Design review of the part built by this model. Coordinates are the model's own, in mm. A direction names the side the tool comes from. Give positions to 0.01 mm unless a question says otherwise; leave off trailing zeros. Order: outer loops, then holes, each group sorted by start corner. A loop starts at its lowest first (then second) coordinate and runs counter-clockwise, first axis right, second up. Notation, with made-up numbers: (-29.75, 77) -> (-23.75, 77) arc R11 cw to (-23.75, 85) -> close; hole circle Ø8 at (15.5, -34.75). An arc over 180 degrees is marked (long way). Use a Markdown table: item, result. Add a question column.
```python
from build123d import *

# Parameters (mm, degrees)
F1_DEPTH       = 250
F3_D           = 3.7973
F3_CSINK_D     = 7.7978
F3_CSINK_ANGLE = 82
F2_W           = 5
F2_H           = 110
F4_DEPTH       = 13.001
F5_R           = 4.99999
F6_T1_DEPTH    = 240.00002
F6_T6_ANGLE    = 359.64
F6_T12_ANGLE   = 359.64


# Not quite as in the source:
# - a fillet or chamfer that OpenCascade refuses, or shapes differently, is made with other operations: its cross-section is extruded or revolved along the edge and cut away or added
# - a fillet or chamfer is up to 0.001 mm smaller than in the source, because OpenCascade refuses the exact size


with BuildPart() as f1:
    # F0 (on Front) → F1 (new body)
    with BuildSketch(Plane.XZ):
        Polygon((-15, 13), (-25, 13), (-25, 0), (0, 0), (0, 3), (-15, 3), align=None)
    extrude(amount=F1_DEPTH)

    # F3 (through all)
    with Locations(Plane(origin=(0, 0, 0), x_dir=(1, 0, 0), z_dir=(0, 0, -1))):
        with Locations((-20, 245), (-20, 125), (-20, 5)):
            CounterSinkHole(F3_D / 2, F3_CSINK_D / 2, counter_sink_angle=F3_CSINK_ANGLE)

    # F2 (on face) → F4 (cut, through all)
    with BuildSketch(Plane(origin=(0, 0, 0), x_dir=(1, 0, 0), z_dir=(0, 0, -1))):
        with Locations((-22.5, 185)):
            Rectangle(F2_W, F2_H)
        with Locations((-22.5, 65)):
            Rectangle(F2_W, F2_H)
    extrude(amount=-F4_DEPTH, mode=Mode.SUBTRACT)

    # F5 (radius 5 in the source; OpenCascade refuses exactly that, so slightly less here)
    f5_edges = [f1.edges().sort_by_distance(p)[0] for p in [
        (-25, 0, 6.5),
        (-25, -10, 6.5),
        (-25, -120, 6.5),
        (-25, -130, 6.5),
        (-25, -240, 6.5),
        (-25, -250, 6.5),
        (-15, -250, 8),
        (0, -250, 1.5),
        (-15, 0, 8),
        (0, 0, 1.5),
    ]]
    fillet(f5_edges, radius=F5_R)

    # F6: chamfer of 4 x 10 on 1 edges, made by hand

    # F6_s2 → F6_t1 (join)
    with BuildSketch(Plane.XZ.offset(4.99999)):
        Polygon((-15, 7), (-5, 3), (-15, 3), align=None)
    extrude(amount=F6_T1_DEPTH)


with BuildPart() as f6_tool4:
    # F6_s5 → F6_t6 (revolve)
    with BuildSketch(Plane(origin=(-0.0322045944, -5.1254529469, 0), x_dir=(0, 0, 1), z_dir=(0.006283144, 0.9999802609, 0))):
        Polygon((7, -14.9681895603), (3, -4.9681895603), (3, -14.9681895603), align=None)
    revolve(axis=Axis((-19.99999, -4.99999, 3), (0, 0, -1)), revolution_arc=F6_T6_ANGLE)

    split(bisect_by=Plane.XZ, keep=Keep.TOP)

    split(bisect_by=Plane.YZ.offset(-20), keep=Keep.TOP)


with BuildPart() as f1_1:
    add(f1.part)

    # F6_t3: union F6_tool4
    add(f6_tool4.part)


with BuildPart() as f6_tool10:
    # F6_s11 → F6_t12 (revolve)
    with BuildSketch(Plane(origin=(1.538550391, -244.8646775786, 0), x_dir=(0, 0, 1), z_dir=(0.006283144, -0.9999802609, 0))):
        Polygon((7, 16.5389755517), (3, 6.5389755517), (3, 16.5389755517), align=None)
    revolve(axis=Axis((-19.99999, -245.00001, 3), (0, 0, 1)), revolution_arc=F6_T12_ANGLE)

    split(bisect_by=Plane.XZ.offset(250), keep=Keep.BOTTOM)

    split(bisect_by=Plane.YZ.offset(-20), keep=Keep.TOP)


with BuildPart() as f1_2:
    add(f1_1.part)

    # F6_t9: union F6_tool10
    add(f6_tool10.part)


solid = f1_2.part
```
1) Machinability: for faces 1 (the flat face through (-10, -123, 0)), 2 (the cylindrical face through (-23, -121, 7)), which of the approach directions +Z, -Z, +X, -X, +Y, -Y give a long, thin tool a straight path to every point of the face, cutting with its end or side? Answer none if there is none.
2) For L1, parallel to Y at x = -20.5, z = 8.75; L2, parallel to Y at x = -21.5, z = 4; L3, parallel to X at y = -93, z = 8.25, list the stretches that pass through material, from the lowest coordinate up. Write a range as [from, to].
3) Insertion check: pin 1 (4 mm diameter, centred on y = -66, z = 6.5, fed in from -X); pin 2 (6 mm diameter, centred on x = -7, y = -80, fed in from +Z); pin 3 (4.5 mm diameter, centred on x = -3, y = -159.5, fed in from +Z). Each pin has a flat end and moves straight along its axis. Give the tip position at first contact, or say it passes through.
4) Add section B-B (y = -165). Give the boundary of the cut face in (x, z).
5) The part is to be moulded in two halves that separate along X. For faces 3 (the cylindrical face through (-2, -249, 2)), 4 (the cylindrical face through (-21.8, -5.6, 7.7)), 5 (the cylindrical face through (-23, -241, 7)), say which applies: +X half, -X half, draft (parallel to the pull), parting line (faces both ways), or undercut.
6) Add section A-A (z = 9.5). Give the number of separate pieces and of enclosed holes in the cut face, then the cut area to 3 significant figures.
Worked answers:
| question | item | result |
|---|---|---|
| 1 | face 1 | -Z, +X, -X, +Y, -Y |
| 1 | face 2 | +Z, -Z, -X |
| 2 | L1 | [-249.97, -246.83], [-243.17, -240.03], [-129.97, -126.83], [-123.17, -120.03], [-9.97, -6.83], [-3.17, -0.03] |
| 2 | L2 | [-249.77, -246.16], [-243.84, -240.23], [-129.77, -126.16], [-123.84, -120.23], [-9.77, -6.16], [-3.84, -0.23] |
| 2 | L3 | [-20, -15] |
| 3 | pin 1 | x = -20 |
| 3 | pin 2 | z = 5 |
| 3 | pin 3 | z = 3.1 |
| 4 | outline | (-20, 0) -> (0, 0) -> (0, 3) -> (-5, 3) -> (-15, 7) -> (-15, 13) -> (-20, 13) -> close |
| 5 | face 3 | +X half |
| 5 | face 4 | undercut |
| 5 | face 5 | -X half |
| 6 | separate pieces | 1 |
| 6 | enclosed holes | 3 |
| 6 | area | 1,320 mm^2 |
